Autodesk Inventor part; units mm, degrees
ref_plane "YZ Plane" through (0, 0, 0) normal (1, 0, 0) x (0, 1, 0)
ref_plane "XZ Plane" through (0, 0, 0) normal (0, 1, 0) x (-1, 0, 0)
ref_plane "XY Plane" through (0, 0, 0) normal (0, 0, 1) x (1, 0, 0)
sketch "DM3D-SF, DX3D-SF_53" plane through (0, 0, 0) normal (0, 0, 1) x (1, 0, 0)
  line L0 (-5.8928, 9.271) -> (7.0612, 9.271)
  line L1 (7.0612, 9.271) -> (7.0612, -3.0988)
  line L2 (7.0612, -3.0988) -> (5.9944, -3.0988)
  line L3 (5.9944, -3.0988) -> (5.6642, -2.794)
  line L4 (5.6642, -2.794) -> (5.6642, -1.1938)
  line L5 (5.6642, -1.1938) -> (-4.4958, -1.1938)
  line L6 (-4.4958, -1.1938) -> (-4.4958, -2.794)
  line L7 (-4.4958, -2.794) -> (-4.8006, -3.0988)
  line L8 (-4.8006, -3.0988) -> (-5.8928, -3.0988)
  line L9 (-5.8928, -3.0988) -> (-5.8928, 9.271)
extrude "Extrusion1" add sketch "DM3D-SF, DX3D-SF_53" along normal blind 6.35
properties part number "DX3D-SF"
Read the model definition and answer for the solid it produces. Units are mm, in the model's axes. A direction names the side the tool comes from. Give positions to 0.01 mm unless a question says otherwise; leave off trailing zeros. Write each loop counter-clockwise with the first axis right and the second up, starting at its lowest first coordinate (ties: lowest second). Pieces come first, ordered by that corner, then holes. Notation, with made-up numbers: M 9,2.25 L 28,2.25 A18 cw 28,14.25 Z; hole C -25.75,72 d11. An arc over 180 degrees is marked long. Put each result on its own line as item: value. Start each with the question number.
1. Consider line 1 along X through (y, z) = (-2.5, 1.5); line 2 along Y through (x, z) = (2.5, 3.5); line 3 along Y through (x, z) = (5.75, 5.5). Determine where each line is inside the solid, lowest interval first.
2. The part is cut by section A-A, the plane y = -2. Give the vertices of the cut face in (x, z).
3. The part is cut by section B-B, the plane z = 3.5. Give the vertices of the cut face in (x, y), and give its area (3 significant figures).
4. The part is cut by section C-C, the plane x = -0.5. Give the vertices of the cut face in (y, z), and give its area (3 significant figures).
5. For a pull along X with two mould halves and no side action, classify faces 1 (the flat face through (5.664, -2, 3)), 2 (the flat face through (-5.893, 3, 3)), 3 (the flat face through (0, 3, 0)) as released by +X, released by -X, zero draft, split by the parting line, or undercut.
6. Which of the six approach directions +Z, -Z, +X, -X, +Y, -Y give full straight-line access (tool end or side, diameter ignored) to faces 4 (the flat face through (6.5, -3.099, 3.1)), 5 (the flat face through (-4.496, -2, 3))?
7. This flat-tipped pin is pushed along its axis until it touches: pin 1 Ø3 at (x, z) = (1.5, 2.5) entering from -Y. Where does it stop, or does it pass through?
Final values:
1. line 1: x = -5.89 to -4.5, 5.66 to 7.06
1. line 2: y = -1.19 to 9.27
1. line 3: y = -2.87 to 9.27
2. outline: M -5.89,0 L -4.5,0 L -4.5,6.35 L -5.89,6.35 Z; M 5.66,0 L 7.06,0 L 7.06,6.35 L 5.66,6.35 Z
3. outline: M -5.89,-3.1 L -4.8,-3.1 L -4.5,-2.79 L -4.5,-1.19 L 5.66,-1.19 L 5.66,-2.79 L 5.99,-3.1 L 7.06,-3.1 L 7.06,9.27 L -5.89,9.27 Z
3. area: 141 mm²
4. outline: M -1.19,0 L 9.27,0 L 9.27,6.35 L -1.19,6.35 Z
4. area: 66.5 mm²
5. face 1: undercut
5. face 2: released by -X
5. face 3: zero draft
6. face 4: +Z, -Z, +X, -X, -Y
6. face 5: +Z, -Z, -Y
7. pin 1: stops at y = -1.19
